Answer from the drawing. Dimensions are ordinates in mm from the lowest x, y and z of the part. Give positions to 0.01 mm unless a question says otherwise; leave off trailing zeros. Write each loop counter-clockwise with the first axis right and the second up, starting at its lowest first coordinate (ties: lowest second). Pieces come first, ordered by that corner, then holes. Notation, with made-up numbers: (-40, -37.5) -> (8, -37.5) arc R27 cw to (8, -5.5) -> close; hole circle Ø9 at (34.5, 49). An arc over 180 degrees is marked (long way). Use a Markdown table: item, result. Add a question column.
Q1. Section A-A, the plane z = 936 is taken. Give the vertices of the cut face in (x, y), plus the area to 3 significant figures.
Q2. For a pull along X with two mould halves and no side action, classify the marked faces 1, 2, 3 and 4 as pulls with the +X half, pulls with the -X half, needs draft (parallel to the pull), parting line crosses it, or undercut.
Q3. Section B-B, the plane y = 295.5 is taken. Give the vertices of the cut face in (x, z).
Q4. Section C-C, the plane z = 500 is taken. Give the vertices of the cut face in (x, y).
Q5. Each of these flat-tipped pins is pushed along its axis until it touches: pin 1 Ø10 at (y, z) = (389.5, 764) entering from -X; pin 2 Ø4 at (x, y) = (372.5, 274.5) entering from +Z; pin 3 Ø2 at (x, z) = (366.5, 641) entering from -Y; pin 4 Ø4 at (x, z) = (1446, 447.5) entering from +Y. Where does it stop, or does it pass through?
Q6. Consider line 1 (X direction, y = 154.5, z = 202); line 2 (Z direction, x = 727.5, y = 506); line 3 (Z direction, x = 87.5, y = 606). Determine where each line is inside the solid, lowest interval first.
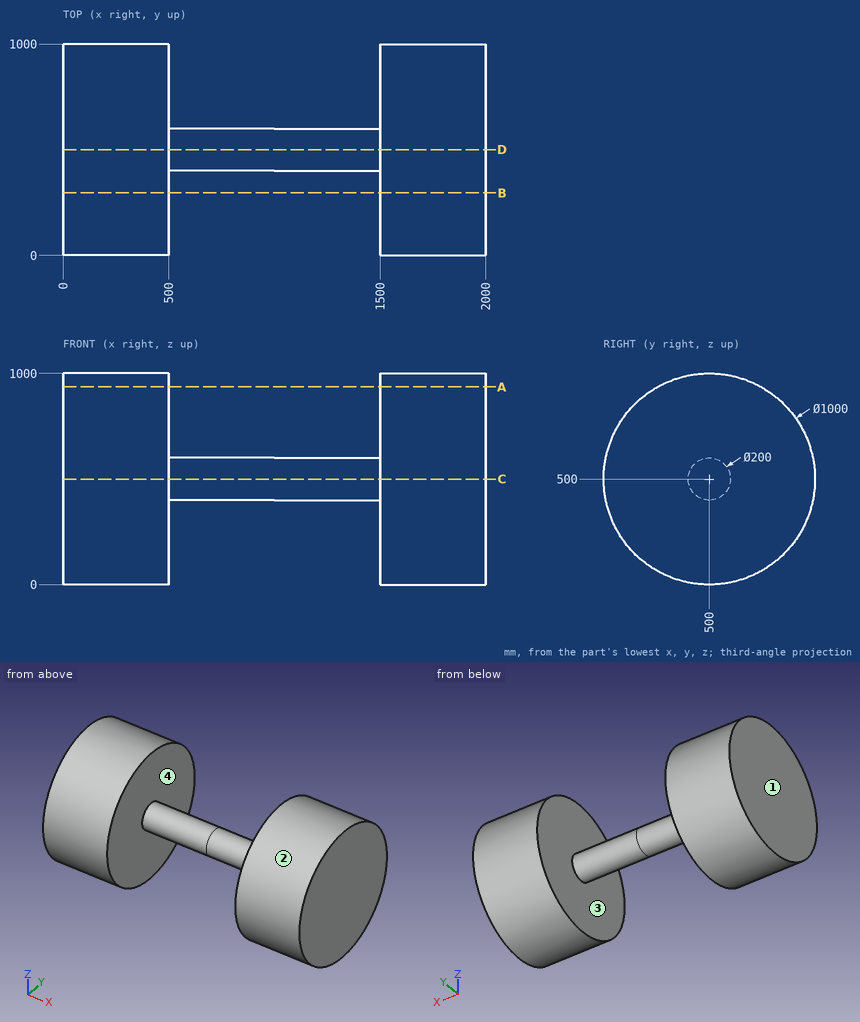
Result set:
| question | item | result |
|---|---|---|
| 1 | outline | (0, 255.25) -> (500, 255.25) -> (500, 744.75) -> (0, 744.75) -> close; (1500, 255.25) -> (2000, 255.25) -> (2000, 744.75) -> (1500, 744.75) -> close |
| 1 | area | 490,000 mm2 |
| 2 | face 1 | pulls with the -X half |
| 2 | face 2 | needs draft |
| 2 | face 3 | undercut |
| 2 | face 4 | undercut |
| 3 | outline | (0, 43.73) -> (500, 43.73) -> (500, 956.27) -> (0, 956.27) -> close; (1500, 43.73) -> (2000, 43.73) -> (2000, 956.27) -> (1500, 956.27) -> close |
| 4 | outline | (0, 0) -> (500, 0) -> (500, 400) -> (1500, 400) -> (1500, 0) -> (2000, 0) -> (2000, 1000) -> (1500, 1000) -> (1500, 600) -> (500, 600) -> (500, 1000) -> (0, 1000) -> close |
| 5 | pin 1 | stops at x = 0 |
| 5 | pin 2 | stops at z = 947.27 |
| 5 | pin 3 | stops at y = 20 |
| 5 | pin 4 | stops at y = 586.31 |
| 6 | line 1 | x = 0 to 500, 1500 to 2000 |
| 6 | line 2 | z = 400.18 to 599.82 |
| 6 | line 3 | z = 11.37 to 988.63 |
